Input: part model. Units: mm. Frame: model coordinates. A direction names the side the tool comes from. Coordinates: 2 decimals unless noted, no trailing zeros. Write each loop counter-clockwise with the first axis right and the second up, starting at its lowest first coordinate (ties: lowest second). Pieces come first, ordered by that corner, then holes. Notation, with made-up numbers: (63.25, -24.5) -> (81.25, -24.5) arc R34 cw to (81.25, 11.5) -> close; hole circle Ø11 at (-33, 87). An arc over 180 degrees is marked (long way). Use one line per item in the form item = value. Start each with the question number.
(1) First-contact query: pin 1 (24 mm diameter, centred on x = -14, y = 10, fed in from +Z). Flat tip, straight axial feed; report the tip coordinate or a pass-through.
(2) Cut plane A-A on z = 8. State how many separate pieces and enclosed holes the cut face has, plus the area to 3 significant figures.
(3) Pull-direction query (X, two-part tool) for faces 4 (the face through (32.7, 37, 5.7)), 5 (the face through (-40, 0.2, 2.6)), 6 (the face through (30, -38, 8)); classes: released by +X, released by -X, zero draft, split by the parting line, or undercut.
(4) Cut plane B-B on x = 35. Return the cut outline in (y, z), plus the area to 3 significant figures.
(5) Set-up query: faces 1 (the face through (-32.47, 38.52, 9.61)), 2 (the face through (-32.8, 37, 5.7)), 3 (the face through (30, 39, 8)). Return all of +Z, -Z, +X, -X, +Y, -Y with unobstructed straight access to the full face (end or side cutting, diameter ignored); none if empty.
(6) Cut plane C-C on y = -15. Return the cut outline in (x, z).
(7) Ray query, line 1 along X through (y, z) = (38.6, 8); line 2 along Z through (x, y) = (35, -39.4); line 3 along Y through (x, z) = (-34, 11.75). Return the intervals inside material, ascending.
```python
from build123d import *

# Parameters (mm, degrees)
SKETCH1_W           = 80
SKETCH1_H           = 80
BOSS_EXTRUDE1_DEPTH = 3
SKETCH9_W           = 10
SKETCH9_H           = 10
SKETCH9_R           = 3
BOSS_EXTRUDE8_DEPTH = 3
BOSS_EXTRUDE9_START = -3
SKETCH10_W          = 10
SKETCH10_H          = 10
SKETCH10_R          = 3
BOSS_EXTRUDE9_DEPTH = 3


with BuildPart() as part:
    # Sketch1 → Boss-Extrude1 (new body)
    with BuildSketch(Plane.XY):
        Rectangle(SKETCH1_W, SKETCH1_H)
    extrude(amount=BOSS_EXTRUDE1_DEPTH)

    # Sketch9 → Boss-Extrude8 (add)
    # profile 1 of 2: a face of its own
    with BuildSketch(Plane(origin=(0, 40, 0), x_dir=(1, 0, 0), z_dir=(0, 1, 0))):
        with Locations((-35, -8)):
            Rectangle(SKETCH9_W, SKETCH9_H)
        with Locations(Location((-35, -8, 0), (0, 0, 270))):
            Circle(SKETCH9_R, mode=Mode.SUBTRACT)
    # profile 2 of 2: a face of its own
    with BuildSketch(Plane(origin=(0, 40, 0), x_dir=(1, 0, 0), z_dir=(0, 1, 0))):
        with Locations((35, -8)):
            Rectangle(SKETCH9_W, SKETCH9_H)
        with Locations(Location((35, -8, 0), (0, 0, 270))):
            Circle(SKETCH9_R, mode=Mode.SUBTRACT)
    extrude(amount=-BOSS_EXTRUDE8_DEPTH)

    # Sketch10 → Boss-Extrude9 (add)
    # profile 1 of 2: a face of its own
    with BuildSketch(Plane.XZ.offset(40).offset(BOSS_EXTRUDE9_START)):
        with Locations((-35, 8)):
            Rectangle(SKETCH10_W, SKETCH10_H)
        with Locations(Location((-35, 8, 0), (0, 0, 90))):
            Circle(SKETCH10_R, mode=Mode.SUBTRACT)
    # profile 2 of 2: a face of its own
    with BuildSketch(Plane.XZ.offset(40).offset(BOSS_EXTRUDE9_START)):
        with Locations((35, 8)):
            Rectangle(SKETCH10_W, SKETCH10_H)
        with Locations(Location((35, 8, 0), (0, 0, 90))):
            Circle(SKETCH10_R, mode=Mode.SUBTRACT)
    extrude(amount=BOSS_EXTRUDE9_DEPTH)


solid = part.part
```
Values:
q1.pin_1 = 3
q2.separate_pieces = 8
q2.enclosed_holes = 0
q2.area = 48.0 mm2
q3.face_4 = zero draft
q3.face_5 = released by -X
q3.face_6 = undercut
q4.outline = (-40, 0) -> (40, 0) -> (40, 5) -> (37, 5) -> (37, 3) -> (-37, 3) -> (-37, 5) -> (-40, 5) -> close; (-40, 11) -> (-37, 11) -> (-37, 13) -> (-40, 13) -> close; (37, 11) -> (40, 11) -> (40, 13) -> (37, 13) -> close
q4.area = 264 mm2
q5.face_1 = +Y, -Y
q5.face_2 = +Z, +X, -X
q5.face_3 = +Z, +Y, -Y
q6.outline = (-40, 0) -> (40, 0) -> (40, 3) -> (-40, 3) -> close
q7.line_1 = -40 to -38, -32 to -30, 30 to 32, 38 to 40
q7.line_2 = 0 to 5, 11 to 13
q7.line_3 = -40 to -37, 37 to 40
